Check sheet for the modelled part. Datum: model origin and axes. Units: mm. A direction names the side the tool comes from. Round coordinates to 2 decimals unless told otherwise and drop trailing zeros. Order: outer loops, then holes, each group sorted by start corner. A loop starts at its lowest first (then second) coordinate and runs counter-clockwise, first axis right, second up.
(1) Sectioned sample at A-A, the plane z = 0. Enter the section's corners in (x, y), and give its area (3 significant figures).
(2) Sectioned sample at D-D, the plane z = 7. Enter the section's corners in (x, y).
(3) Sectioned sample at B-B, the plane x = 0. Enter the section's corners in (y, z).
(4) Mould release check, pull along Z, two halves, no side actions. Record for faces 1 (the cylindrical face through (0.66, 16.818, -14.985)), 2 (the cylindrical face through (3.755, 14.79, 11.923)), 3 (the flat face through (12.3, 30, -3.4)): released by +Z, released by -Z, zero draft, split by the parting line, or undercut.
(5) Sectioned sample at C-C, the plane x = 18. Enter the section's corners in (y, z), and give its area (3 significant figures).
(6) Thickness scan on probe 1 along X at (y, z) = (2.85, 0); probe 2 along X at (y, z) = (15.25, 0); probe 3 along Y at (x, z) = (-12.5, 17.5). Record the ranges inside material, lowest first.
(7) Tool access check on faces 4 (the flat face through (-15, 4, 5)), 5 (the cylindrical face through (-16.735, 1.972, -0.806)). Record the directions out of +Z, -Z, +X, -X, +Y, -Y that give a thin tool (end or side, any length) a straight path to the whole face; none if there is none.
(8) Depth check by flat-ended pin: pin 1 (5 mm diameter, centred on x = -1, y = 17.5, fed in from +Z); pin 2 (4 mm diameter, centred on x = 0, z = -18, fed in from +Y); pin 3 (1.8 mm diameter, centred on x = 0, z = 18, fed in from -Y); pin 4 (8 mm diameter, centred on x = -16, y = 23, fed in from +Z). Enter the tip coordinate at first touch or a pass-through.
```python
from build123d import *

# Parameters (mm, degrees)
SKETCH_1_R          = 15
SKETCH_1_R_2        = 12.5
EXTRUDE_1_DEPTH     = 30
SKETCH_1_3_R        = 23
SKETCH_1_3_R_2      = 15
EXTRUDE_2_DEPTH     = 4
CUT_EXTRUDE_3_REACH = 46.249
SKETCH_3_R          = 1.5


with BuildPart() as part:
    # Sketch 1 → Extrude 1 (new body)
    with BuildSketch(Plane(origin=(0, 0, 0), x_dir=(1, 0, 0), z_dir=(0, 1, 0))):
        with Locations(Location((0, 0, 0), (0, 0, 270))):
            Circle(SKETCH_1_R)
        with Locations(Location((0, 0, 0), (0, 0, 270))):
            Circle(SKETCH_1_R_2, mode=Mode.SUBTRACT)
    extrude(amount=EXTRUDE_1_DEPTH)

    # Sketch 1_3 → Extrude 2 (add)
    with BuildSketch(Plane(origin=(0, 0, 0), x_dir=(1, 0, 0), z_dir=(0, 1, 0))):
        with Locations(Location((0, 0, 0), (0, 0, 270))):
            Circle(SKETCH_1_3_R)
        with Locations(Location((0, 0, 0), (0, 0, 270))):
            Circle(SKETCH_1_3_R_2, mode=Mode.SUBTRACT)
    extrude(amount=EXTRUDE_2_DEPTH)

    # Sketch 3 → Cut-Extrude 3 (cut, up to next)
    with BuildSketch(Plane.XZ, mode=Mode.PRIVATE) as cut_extrude_3_sk1:
        with Locations(Location((0, 18, 0), (0, 0, 270))):
            Circle(SKETCH_3_R)
    cut_extrude_3_tool1 = extrude(cut_extrude_3_sk1.sketch, amount=-CUT_EXTRUDE_3_REACH, mode=Mode.PRIVATE) & part.part
    # Sketch 3 → Cut-Extrude 3 (cut, up to next)
    with BuildSketch(Plane.XZ, mode=Mode.PRIVATE) as cut_extrude_3_sk2:
        with Locations(Location((18, 0, 0), (0, 0, 270))):
            Circle(SKETCH_3_R)
    cut_extrude_3_tool2 = extrude(cut_extrude_3_sk2.sketch, amount=-CUT_EXTRUDE_3_REACH, mode=Mode.PRIVATE) & part.part
    # Sketch 3 → Cut-Extrude 3 (cut, up to next)
    with BuildSketch(Plane.XZ, mode=Mode.PRIVATE) as cut_extrude_3_sk3:
        with Locations(Location((0, -18, 0), (0, 0, 270))):
            Circle(SKETCH_3_R)
    cut_extrude_3_tool3 = extrude(cut_extrude_3_sk3.sketch, amount=-CUT_EXTRUDE_3_REACH, mode=Mode.PRIVATE) & part.part
    # Sketch 3 → Cut-Extrude 3 (cut, up to next)
    with BuildSketch(Plane.XZ, mode=Mode.PRIVATE) as cut_extrude_3_sk4:
        with Locations(Location((-18, 0, 0), (0, 0, 270))):
            Circle(SKETCH_3_R)
    cut_extrude_3_tool4 = extrude(cut_extrude_3_sk4.sketch, amount=-CUT_EXTRUDE_3_REACH, mode=Mode.PRIVATE) & part.part
    add(cut_extrude_3_tool1.solids().sort_by_distance((0, 0, 18))[0], mode=Mode.SUBTRACT)
    add(cut_extrude_3_tool2.solids().sort_by_distance((18, 0, 0))[0], mode=Mode.SUBTRACT)
    add(cut_extrude_3_tool3.solids().sort_by_distance((0, 0, -18))[0], mode=Mode.SUBTRACT)
    add(cut_extrude_3_tool4.solids().sort_by_distance((-18, 0, 0))[0], mode=Mode.SUBTRACT)


solid = part.part
```
Derived:
1. outline: (-23, 0) - (-19.5, 0) - (-19.5, 4) - (-23, 4) - close; (-16.5, 0) - (-12.5, 0) - (-12.5, 30) - (-15, 30) - (-15, 4) - (-16.5, 4) - close; (12.5, 0) - (16.5, 0) - (16.5, 4) - (15, 4) - (15, 30) - (12.5, 30) - close; (19.5, 0) - (23, 0) - (23, 4) - (19.5, 4) - close
1. area: 190 mm2
2. outline: (-21.91, 0) - (-10.36, 0) - (-10.36, 30) - (-13.27, 30) - (-13.27, 4) - (-21.91, 4) - close; (10.36, 0) - (21.91, 0) - (21.91, 4) - (13.27, 4) - (13.27, 30) - (10.36, 30) - close
3. outline: (0, -23) - (4, -23) - (4, -19.5) - (0, -19.5) - close; (0, -16.5) - (4, -16.5) - (4, -15) - (30, -15) - (30, -12.5) - (0, -12.5) - close; (0, 12.5) - (30, 12.5) - (30, 15) - (4, 15) - (4, 16.5) - (0, 16.5) - close; (0, 19.5) - (4, 19.5) - (4, 23) - (0, 23) - close
4. face 1: split by the parting line
4. face 2: undercut
4. face 3: zero draft
5. outline: (0, -14.32) - (4, -14.32) - (4, -1.5) - (0, -1.5) - close; (0, 1.5) - (4, 1.5) - (4, 14.32) - (0, 14.32) - close
5. area: 103 mm2
6. probe 1: x = -23 to -19.5, -16.5 to -12.5, 12.5 to 16.5, 19.5 to 23
6. probe 2: x = -15 to -12.5, 12.5 to 15
6. probe 3: y = 0 to 4
7. face 4: +Y
7. face 5: +Y, -Y
8. pin 1: stops at z = 15
8. pin 2: stops at y = 4
8. pin 3: passes through
8. pin 4: stops at z = 9
